```python
from build123d import *

# Parameters (mm, degrees)
SKETCH1_W           = 82.804
SKETCH1_H           = 31.75
BOSS_EXTRUDE1_DEPTH = 3.175
SKETCH2_W           = 3.2258
SKETCH2_H           = 6.35
CUT_FOR_TAB_DEPTH   = 4.175
CUT_EXTRUDE1_DEPTH  = 4.175


with BuildPart() as part:
    # Sketch1 → Boss-Extrude1 (new body)
    with BuildSketch(Plane.XY):
        Rectangle(SKETCH1_W, SKETCH1_H)
    extrude(amount=BOSS_EXTRUDE1_DEPTH)

    # Sketch2 → cut for tab (cut, through all)
    with BuildSketch(Plane.XY.offset(3.175)):
        with Locations((-36.6141, 6.35)):
            Rectangle(SKETCH2_W, SKETCH2_H)
        with Locations((-36.6141, -6.35)):
            Rectangle(SKETCH2_W, SKETCH2_H)
    cut_for_tab = extrude(amount=-CUT_FOR_TAB_DEPTH, mode=Mode.SUBTRACT)

    # Mirror1: cut for tab across plane
    add(cut_for_tab.mirror(Plane(origin=(0, 0, 0), x_dir=(0, 0, 1), z_dir=(1, 0, 0))), mode=Mode.SUBTRACT)

    # Sketch3 → Cut-Extrude1 (cut, through all)
    with BuildSketch(Plane.XY.offset(3.175)):
        Polygon((0, 15.875), (0, 9.525), (-25.4, 9.525), (-31.75, 15.875), align=None)
    cut_extrude1 = extrude(amount=-CUT_EXTRUDE1_DEPTH, mode=Mode.SUBTRACT)

    # Mirror2: Cut-Extrude1 across plane
    add(cut_extrude1.mirror(Plane(origin=(0, 0, 0), x_dir=(0, 0, 1), z_dir=(1, 0, 0))), mode=Mode.SUBTRACT)


solid = part.part
```
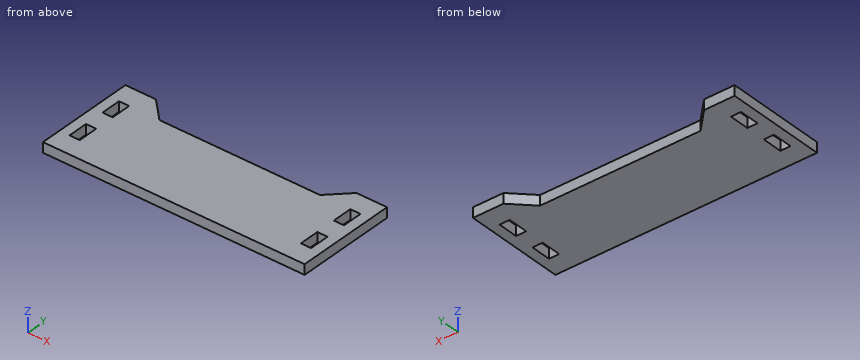
Input: part model. Units: mm. Frame: model coordinates. Coordinates: 2 decimals unless noted, no trailing zeros. Write each loop counter-clockwise with the first axis right and the second up, starting at its lowest first coordinate (ties: lowest second). Pieces come first, ordered by that corner, then holes. Notation, with made-up numbers: M 89.25,-29.5 L 147.25,-29.5 A8 cw 147.25,-16.5 Z; hole C 23,83 d1. An arc over 180 degrees is marked long. Use one line per item in the form item = value.
Q1. Section B-B (z = 1.6). Return loops of the section in (x, y) (3 decimals), plus the area to 3 significant figures.
Answer below:
outline = M -41.402,-15.875 L 41.402,-15.875 L 41.402,15.875 L 31.75,15.875 L 25.4,9.525 L -25.4,9.525 L -31.75,15.875 L -41.402,15.875 Z; hole M -38.227,-9.525 L -35.001,-9.525 L -35.001,-3.175 L -38.227,-3.175 Z; hole M -38.227,3.175 L -35.001,3.175 L -35.001,9.525 L -38.227,9.525 Z; hole M 35.001,-9.525 L 38.227,-9.525 L 38.227,-3.175 L 35.001,-3.175 Z; hole M 35.001,3.175 L 38.227,3.175 L 38.227,9.525 L 35.001,9.525 Z
area = 2,180 mm²
Q2. Section D-D (x = -7). Return loops of the section in (y, z) (3 decimals).
Answer below:
outline = M -15.875,0 L 9.525,0 L 9.525,3.175 L -15.875,3.175 Z
Q3. Material intervals for probe 1 along X at (y, z) = (4, 1.2); probe 2 along Y at (x, z) = (21.5, 1.65) (3 decimals); probe 3 along X at (y, z) = (14.5, 0.3) (3 decimals), sorted ascending. Write a range as from..to.
Answer below:
probe_1 = -41.4..-38.23, -35..35, 38.23..41.4
probe_2 = -15.875..9.525
probe_3 = -41.402..-30.375, 30.375..41.402
Q4. Section C-C (y = 12). Return loops of the section in (x, z) (3 decimals), plus the area to 3 significant figures.
Answer below:
outline = M -41.402,0 L -27.875,0 L -27.875,3.175 L -41.402,3.175 Z; M 27.875,0 L 41.402,0 L 41.402,3.175 L 27.875,3.175 Z
area = 85.9 mm²
Q5. First-contact query: pin 1 (1.6 mm diameter, centred on x = -2.5, z = 2, fed in from +Y) (3 decimals). Flat tip, straight axial feed; report the tip coordinate or a pass-through.
Answer below:
pin_1 = 9.525
Q6. Section A-A (y = 8). Return loops of the section in (x, z) (3 decimals).
Answer below:
outline = M -41.402,0 L -38.227,0 L -38.227,3.175 L -41.402,3.175 Z; M -35.001,0 L 35.001,0 L 35.001,3.175 L -35.001,3.175 Z; M 38.227,0 L 41.402,0 L 41.402,3.175 L 38.227,3.175 Z
